Check sheet for the drawn part. Datum: minimum x, y, z corner. Units: mm. A direction names the side the tool comes from. Give positions to 0.01 mm unless a question says otherwise; leave off trailing zeros. Write each loop counter-clockwise with the first axis right and the second up, starting at its lowest first coordinate (ties: lowest second). Pieces come first, ordered by that corner, then holes.
(1) Tool access check on the marked faces 1, 2, 3 and 4. Record the directions out of +Z, -Z, +X, -X, +Y, -Y that give a thin tool (end or side, any length) a straight path to the whole face; none if there is none.
(2) Cross-section at C-C (x = 17). Record the boundary of the cut face in (y, z).
(3) Thickness scan on line 1 along Z through (x, y) = (5.5, 33.6); line 2 along Z through (x, y) = (5, 34); line 3 along X through (y, z) = (34.45, 45). Record the ranges inside material, lowest first.
(4) Cross-section at A-A (x = 54.5). Record the boundary of the cut face in (y, z), and give its area (3 significant figures).
(5) Cross-section at D-D (y = 18.5). Record the boundary of the cut face in (x, z).
(6) Cross-section at B-B (z = 45). Record the boundary of the cut face in (x, y), and give its area (3 significant figures).
(7) Depth check by flat-ended pin: P1, Ø2, axis at y = 34.5, z = 44.5, coming from the -X side; P2, Ø1.6, axis at y = 34.5, z = 48.5, coming from the +X side; P3, Ø1.5, axis at x = 10.5, z = 39.5, coming from the -Y side; P4, Ø2.5, axis at x = 6.5, z = 46, coming from the +Y side. Enter the tip coordinate at first touch or a pass-through.
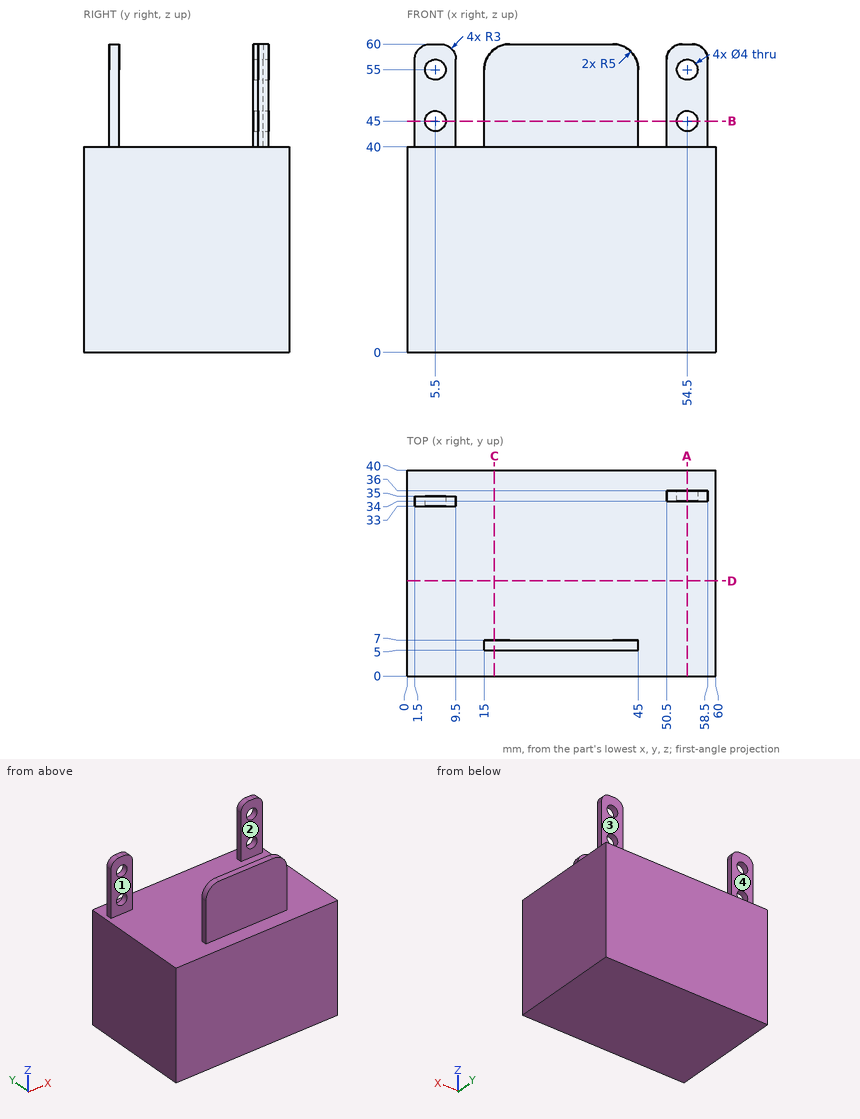
Reply:
1. face 1: +Z, +X, -X, -Y
1. face 2: +Z, +X, -Y
1. face 3: +Z, +X, -X, +Y
1. face 4: +Z, -X, +Y
2. outline: (0, 0) - (40, 0) - (40, 40) - (7, 40) - (7, 59) - (5, 59) - (5, 40) - (0, 40) - close
3. line 1: z = 0 to 43, 47 to 53, 57 to 60
3. line 2: z = 0 to 43.06, 46.94 to 53.06, 56.94 to 60
3. line 3: x = 1.5 to 3.5, 7.5 to 9.5, 50.5 to 52.5, 56.5 to 58.5
4. outline: (0, 0) - (40, 0) - (40, 40) - (36, 40) - (36, 43) - (34, 43) - (34, 40) - (0, 40) - close; (34, 47) - (36, 47) - (36, 53) - (34, 53) - close; (34, 57) - (36, 57) - (36, 60) - (34, 60) - close
4. area: 1,620 mm2
5. outline: (0, 0) - (60, 0) - (60, 40) - (0, 40) - close
6. outline: (1.5, 33) - (3.5, 33) - (3.5, 35) - (1.5, 35) - close; (7.5, 33) - (9.5, 33) - (9.5, 35) - (7.5, 35) - close; (15, 5) - (45, 5) - (45, 7) - (15, 7) - close; (50.5, 34) - (52.5, 34) - (52.5, 36) - (50.5, 36) - close; (56.5, 34) - (58.5, 34) - (58.5, 36) - (56.5, 36) - close
6. area: 76.0 mm2
7. P1: stops at x = 1.5
7. P2: stops at x = 58.5
7. P3: stops at y = 0
7. P4: stops at y = 35
